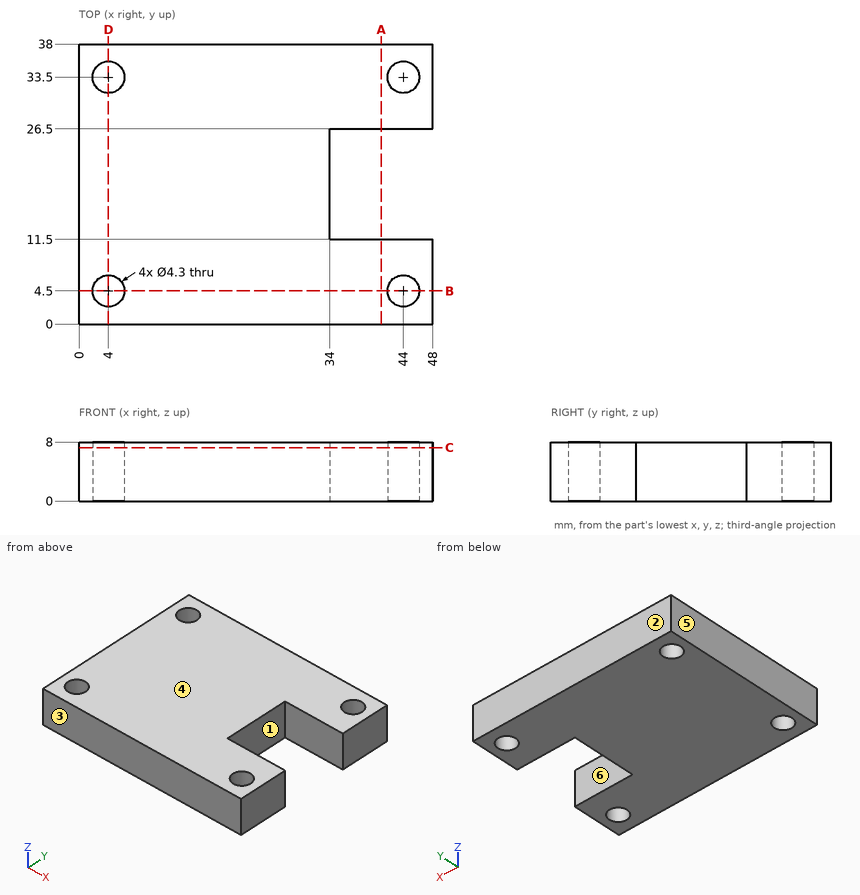
Verification items for this drawing (mm, ordinates from the low corner). A direction names the side the tool comes from. Coordinates: 2 decimals unless noted, no trailing zeros. Loops run counter-clockwise (first coordinate to the right, second up) from the corner with the lowest first, then second, coordinate; pieces in that order, holes last. Notation, with made-up numbers: (71.5, 31) - (115.5, 31) arc R31 ccw to (115.5, 60) - close; hole circle Ø5 at (76.25, 61). An arc over 180 degrees is marked (long way). Use one line per item in the form item = value. Start each with the question number.
Item 1: Mould release check, pull along Y, two halves, no side actions. Record for the marked faces 1, 2, 3 and 4: +Y half, -Y half, draft (parallel to the pull), parting line (faces both ways), or undercut.
Item 2: Gauge pin test, flat end, axial feed: pin 1 (4 mm diameter, centred on y = 21.5, z = 3, fed in from +X). Record the tip position at first contact, or that the pin passes through.
Item 3: Section check D-D, the plane x = 4. Enter the section's corners in (y, z), and give its area (3 significant figures).
Item 4: Section check B-B, the plane y = 4.5. Enter the section's corners in (x, z).
Item 5: Tool access check on the marked faces 5 and 6. Record the directions out of +Z, -Z, +X, -X, +Y, -Y that give a thin tool (end or side, any length) a straight path to the whole face; none if there is none.
Item 6: Section check A-A, the plane x = 41. Enter the section's corners in (y, z), and give its area (3 significant figures).
Item 7: Thickness scan on probe 1 along Y at (x, z) = (44, 2.75); probe 2 along Y at (x, z) = (4, 5); probe 3 along Y at (x, z) = (41, 4.75). Record the ranges inside material, lowest first.
Item 8: Section check C-C, the plane z = 7.25. Enter the section's corners in (x, y), and give its area (3 significant figures).
Computed:
q1.face_1 = undercut
q1.face_2 = +Y half
q1.face_3 = -Y half
q1.face_4 = draft
q2.pin_1 = 34
q3.outline = (0, 0) - (2.35, 0) - (2.35, 8) - (0, 8) - close; (6.65, 0) - (31.35, 0) - (31.35, 8) - (6.65, 8) - close; (35.65, 0) - (38, 0) - (38, 8) - (35.65, 8) - close
q3.area = 235 mm2
q4.outline = (0, 0) - (1.85, 0) - (1.85, 8) - (0, 8) - close; (6.15, 0) - (41.85, 0) - (41.85, 8) - (6.15, 8) - close; (46.15, 0) - (48, 0) - (48, 8) - (46.15, 8) - close
q5.face_5 = +Z, -Z, -X, +Y, -Y
q5.face_6 = +Z, -Z, +X
q6.outline = (0, 0) - (11.5, 0) - (11.5, 8) - (0, 8) - close; (26.5, 0) - (38, 0) - (38, 8) - (26.5, 8) - close
q6.area = 184 mm2
q7.probe_1 = 0 to 2.35, 6.65 to 11.5, 26.5 to 31.35, 35.65 to 38
q7.probe_2 = 0 to 2.35, 6.65 to 31.35, 35.65 to 38
q7.probe_3 = 0 to 11.5, 26.5 to 38
q8.outline = (0, 0) - (48, 0) - (48, 11.5) - (34, 11.5) - (34, 26.5) - (48, 26.5) - (48, 38) - (0, 38) - close; hole circle Ø4.3 at (4, 4.5); hole circle Ø4.3 at (4, 33.5); hole circle Ø4.3 at (44, 4.5); hole circle Ø4.3 at (44, 33.5)
q8.area = 1,560 mm2
